from build123d import *

# Parameters (mm, degrees)
F0_W      = 94
F0_H      = 18.5
F0_W_2    = 75.25
F0_H_2    = 10.5
F2_DEPTH  = 50
F1_W      = 75.25
F1_H      = 10.5
F3_DEPTH  = 20
F4_W      = 11
F4_H      = 7.5
F4_R      = 1.75
F5_DEPTH  = 11
F6_DEPTH  = 27.1777510643
F8_DEPTH  = 8.9369788766
F4_R_2    = 1.8
F9_DEPTH  = 25
F4_R_3    = 3.55
F10_DEPTH = 2.8


with BuildPart() as f2:
    # F0 (on Front) → F2 (new body)
    with BuildSketch(Plane.XZ):
        with Locations((-1.8079760883, 22.0405235887)):
            Rectangle(F0_W, F0_H)
        with Locations((-1.8079760883, 22.0405235887)):
            Rectangle(F0_W_2, F0_H_2, mode=Mode.SUBTRACT)
    extrude(amount=F2_DEPTH)

    # F1 (on face) → F3 (join)
    with BuildSketch(Plane.XZ):
        with Locations((-1.8079760883, 22.0405235887)):
            Rectangle(F1_W, F1_H)
    extrude(amount=F3_DEPTH)

    # F4 (on face) → F5 (cut)
    with BuildSketch(Plane.XZ.offset(20)):
        with Locations((-1.8079760883, 22.0405235887)):
            Rectangle(F4_W, F4_H)
        with Locations((-1.8079760883, 22.0405235887)):
            Circle(F4_R, mode=Mode.SUBTRACT)
    extrude(amount=-F5_DEPTH, mode=Mode.SUBTRACT)

    # F6 (cut): a face of the model
    f6_faces = [f2.faces().sort_by_distance(p)[0] for p in [
        (-1.8079760883, -20, 22.0405235887),
    ]]
    extrude(f6_faces, amount=-F6_DEPTH, mode=Mode.SUBTRACT)

    # F7 (on face) → F8 (cut)
    with BuildSketch(Plane(origin=(0, 0, 12.7905235887), x_dir=(1, 0, 0), z_dir=(0, 0, -1))):
        Polygon((-3.6079760883, 50), (-3.6079760883, 25), (-3.6079760883, 0), (-0.0079760883, 0), (-0.0079760883, 25), (-0.0079760883, 50), (-1.8079760883, 50), align=None)
    extrude(amount=-F8_DEPTH, mode=Mode.SUBTRACT)

    # F4 (on face) → F9 (cut)
    with BuildSketch(Plane.XZ.offset(20)):
        with Locations((-29.3346382678, 22.0405235887)):
            Circle(F4_R_2)
        with Locations((28.2589178532, 22.0405235887)):
            Circle(F4_R_2)
    extrude(amount=-F9_DEPTH, mode=Mode.SUBTRACT)

    # F4 (on face) → F10 (cut)
    with BuildSketch(Plane.XZ.offset(20)):
        with Locations((28.2589178532, 22.0405235887)):
            Circle(F4_R_3)
        with Locations((28.2589178532, 22.0405235887)):
            Circle(F4_R_2, mode=Mode.SUBTRACT)
        with Locations((-29.3346382678, 22.0405235887)):
            Circle(F4_R_3)
        with Locations((-29.3346382678, 22.0405235887)):
            Circle(F4_R_2, mode=Mode.SUBTRACT)
    extrude(amount=-F10_DEPTH, mode=Mode.SUBTRACT)


solid = f2.part
Here's how the part is built. I have some questions about the finished solid (model axes, mm). A direction names the side the tool comes from. Give positions to 0.01 mm unless a question says otherwise; leave off trailing zeros. Write each loop counter-clockwise with the first axis right and the second up, starting at its lowest first coordinate (ties: lowest second). Pieces come first, ordered by that corner, then holes. Notation, with made-up numbers: (6.25, 64) -> (55.25, 64) arc R22 ccw to (55.25, 100) -> close; hole circle Ø8 at (70.25, 84). An arc over 180 degrees is marked (long way). Use one line per item in the form item = value. Start each with the question number.
1. If I drill on L1, parallel to Z at x = 13, y = -34; L2, parallel to X at y = -33, z = 25.75; L3, parallel to X at y = -5, z = 22, over which ranges is the centre line in solid material (lowest first)?
2. On a 3-axis mill with a long thin cutter (end or side, diameter ignored), from which of +Z, -Z, +X, -X, +Y, -Y can I reach the whole of each face in a straight line? I mean faces 1 (the face through (-0.008, -19, 16)), 2 (the face through (-2, -50, 28)), 3 (the face through (-3, -9, 24)). Say none if no direction works.
3. Will these pins go through, and if not, where does the flat tip stop? pin 1 Ø2 at (x, z) = (26.5, 23.5) entering from -Y; pin 2 Ø3 at (x, z) = (-16, 21.5) entering from -Y.
4. Imagine slicing it at C-C on y = -37. List the corners of the cut face in (x, z) for me.
5. Imagine slicing it at A-A on z = 15.75. List the corners of the cut face in (x, y) for me, plus the area to 3 significant figures.
6. Imagine slicing it at B-B on x = 28. List the corners of the cut face in (y, z) for me.
7. Thinking about a two-plate mould opening in Z: for faces 4 (the face through (-48.808, -25, 22)), 5 (the face through (-22, -35, 16.791)), 6 (the face through (-2, -25, 31.291)), which applies, +Z half, -Z half, draft (parallel to the pull), parting line (faces both ways), or undercut?
8. Imagine slicing it at D-D on x = -24.5. List the corners of the cut face in (y, z) for me.
Entries:
q1.L1 = 12.79 to 16.79, 27.29 to 31.29
q1.L2 = -48.81 to -39.43, 35.82 to 45.19
q1.L3 = -48.81 to -31.13, -27.54 to -3.56, -0.06 to 26.46, 30.06 to 45.19
q2.face_1 = -Z, +Y, -Y
q2.face_2 = +Z, -Z, +X, -X, -Y
q2.face_3 = -Y
q3.pin_1 = -17.2
q3.pin_2 = -20
q4.outline = (-48.81, 12.79) -> (-3.61, 12.79) -> (-3.61, 16.79) -> (-39.43, 16.79) -> (-39.43, 27.29) -> (35.82, 27.29) -> (35.82, 16.79) -> (-0.01, 16.79) -> (-0.01, 12.79) -> (45.19, 12.79) -> (45.19, 31.29) -> (-48.81, 31.29) -> close
q5.outline = (-48.81, -50) -> (-3.61, -50) -> (-3.61, 0) -> (-48.81, 0) -> close; (-0.01, -50) -> (45.19, -50) -> (45.19, 0) -> (-0.01, 0) -> close
q5.area = 4,520 mm²
q6.outline = (-50, 12.79) -> (0, 12.79) -> (0, 20.26) -> (-17.2, 20.26) -> (-17.2, 18.5) -> (-20, 18.5) -> (-20, 16.79) -> (-50, 16.79) -> close; (-50, 27.29) -> (-20, 27.29) -> (-20, 25.58) -> (-17.2, 25.58) -> (-17.2, 23.82) -> (0, 23.82) -> (0, 31.29) -> (-50, 31.29) -> close
q7.face_4 = draft
q7.face_5 = undercut
q7.face_6 = +Z half
q8.outline = (-50, 12.79) -> (0, 12.79) -> (0, 31.29) -> (-50, 31.29) -> (-50, 27.29) -> (-20, 27.29) -> (-20, 16.79) -> (-50, 16.79) -> close
